CAD build for the part. Positions are in the model's coordinates, mm. Face numbers are marked on the shaded views. Give positions to 0.01 mm unless a question says otherwise; leave off trailing zeros. Write each loop counter-clockwise with the first axis right and the second up, starting at its lowest first coordinate (ties: lowest second). Pieces come first, ordered by that corner, then holes. Notation, with made-up numbers: (31.25, 7) - (83.25, 7) arc R20 cw to (83.25, 41) - close; hole circle Ø8 at (3.5, 81). An arc over 180 degrees is marked (long way). Answer as a JSON object with one key per item and string values.
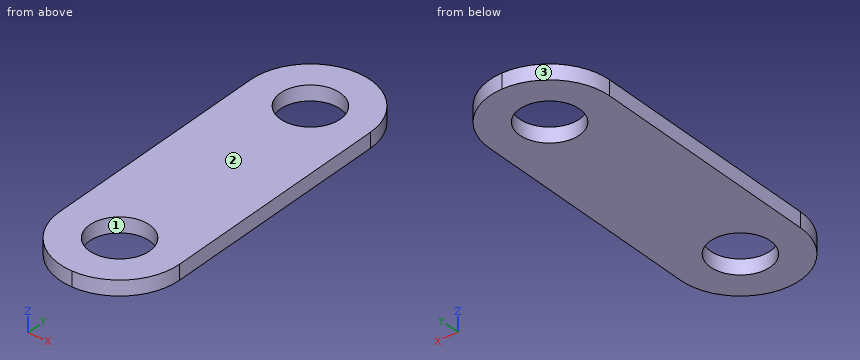
from build123d import *

# Parameters (mm, degrees)
SKETCH1_W           = 12.7
SKETCH1_H           = 38.1
SKETCH1_R           = 3.175
BOSS_EXTRUDE1_DEPTH = 1.5875
FILLET1_R           = 6.35


with BuildPart() as part:
    # Sketch1 → Boss-Extrude1 (new body)
    with BuildSketch(Plane.XY):
        with Locations((6.35, 19.05)):
            Rectangle(SKETCH1_W, SKETCH1_H)
        with Locations((6.35, 31.75)):
            Circle(SKETCH1_R, mode=Mode.SUBTRACT)
        with Locations((6.35, 6.35)):
            Circle(SKETCH1_R, mode=Mode.SUBTRACT)
    extrude(amount=BOSS_EXTRUDE1_DEPTH)

    # Fillet1
    fillet1_edges = [part.edges().sort_by_distance(p)[0] for p in [
        (12.7, 38.1, 0.79375),
        (0, 38.1, 0.79375),
        (0, 0, 0.79375),
        (12.7, 0, 0.79375),
    ]]
    fillet(fillet1_edges, radius=FILLET1_R - 0.0001)  # a hair under: the kernel refuses the full size


solid = part.part
Item 1: Flat gauge pin, fed straight in: P1, Ø4, axis at x = 6.35, y = 31.75, coming from the -Z side. Where does the tip first touch, or does it go through?
Entries:
{"P1": "through"}
Item 2: Mould opens along X. For the marked faces 1, 2 and 3 say: +X half, -X half, draft (parallel to the pull), parting line (faces both ways), or undercut.
Entries:
{"face 1": "undercut", "face 2": "draft", "face 3": "-X half"}
Item 3: Cut at B-B (z = 1). State how many separate pieces and enclosed holes the cut face has, and give its area (3 significant figures).
Entries:
{"separate pieces": "1", "enclosed holes": "2", "area": "386 mm2"}
Item 4: Cut at C-C (x = 8.25). Give the cut face in (y, z), and give its area (3 significant figures).
Entries:
{"outline": "(0.29, 0) - (3.81, 0) - (3.81, 1.59) - (0.29, 1.59) - close; (8.89, 0) - (29.21, 0) - (29.21, 1.59) - (8.89, 1.59) - close; (34.29, 0) - (37.81, 0) - (37.81, 1.59) - (34.29, 1.59) - close", "area": "43.4 mm2"}
Item 5: Probe line 1 (Y direction, x = 6.35, z = 0.7) (3 decimals); line 2 (Y direction, x = 3.75, z = 0.3); line 3 (Y direction, x = 11.5, z = 0.2). List the from-to ranges inside material, lowest first. Write a range as from..to.
Entries:
{"line 1": "0..3.175, 9.525..28.575, 34.925..38.1", "line 2": "0.56..4.53, 8.17..29.93, 33.57..37.54", "line 3": "2.64..35.46"}
Item 6: Cut at A-A (x = 3.75). Give the cut face in (y, z), and give its area (3 significant figures).
Entries:
{"outline": "(0.56, 0) - (4.53, 0) - (4.53, 1.59) - (0.56, 1.59) - close; (8.17, 0) - (29.93, 0) - (29.93, 1.59) - (8.17, 1.59) - close; (33.57, 0) - (37.54, 0) - (37.54, 1.59) - (33.57, 1.59) - close", "area": "47.1 mm2"}
Item 7: Cut at D-D (x = 2.25). Give the cut face in (y, z), and give its area (3 significant figures).
Entries:
{"outline": "(1.5, 0) - (36.6, 0) - (36.6, 1.59) - (1.5, 1.59) - close", "area": "55.7 mm2"}
